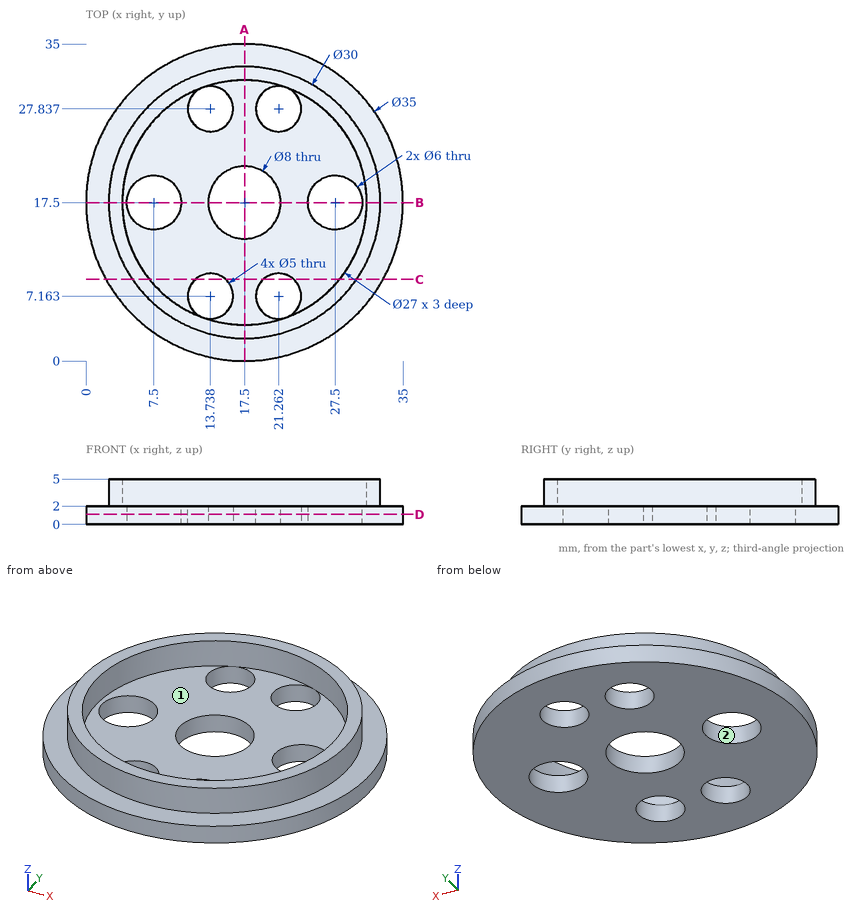
Design review of the part shown in the three views and the two pictorial views. Dimensions are in mm from the part's minimum x, y and z. A direction names the side the tool comes from. Round coordinates to 2 decimals unless told otherwise and drop trailing zeros. Loops run counter-clockwise (first coordinate to the right, second up) from the corner with the lowest first, then second, coordinate; pieces in that order, holes last. Notation, with made-up numbers: M -10,-19.5 L 23,-19.5 A37 ccw 23,17.5 Z; hole C 24,28.25 d5. An arc over 180 degrees is marked long. Answer as a JSON object with one key per item and string values.
Item 1: We need section D-D on z = 1.1. Give the boundary of the cut face in (x, y).
Answer sheet:
{"outline": "C 17.5,17.5 d35; hole C 7.5,17.5 d6; hole C 13.74,7.16 d5; hole C 13.74,27.84 d5; hole C 17.5,17.5 d8; hole C 21.26,7.16 d5; hole C 21.26,27.84 d5; hole C 27.5,17.5 d6"}
Item 2: Wall thickness on L1, parallel to X at y = 27, z = 0.65 (1 decimal); L2, parallel to Y at x = 22.5, z = 1.95 (1 decimal); L3, parallel to X at y = 7.5, z = 0.3 (1 decimal): over which ranges is each line inside the solid? List them lowest first. Write a range as from..to.
Answer sheet:
{"L1": "x = 2.8..11.4, 16.1..18.9, 23.6..32.2", "L2": "y = 0.7..5, 9.3..25.7, 30..34.3", "L3": "x = 3.1..11.3, 16.2..18.8, 23.7..31.9"}
Item 3: Machinability: for the marked faces 1 and 2, which of the approach directions +Z, -Z, +X, -X, +Y, -Y give a long, thin tool a straight path to every point of the face, cutting with its end or side? Answer none if there is none.
Answer sheet:
{"face 1": "+Z", "face 2": "+Z, -Z"}
Item 4: We need section B-B on y = 17.5. Give the boundary of the cut face in (x, z), and give its area (3 significant figures).
Answer sheet:
{"outline": "M 0,0 L 4.5,0 L 4.5,2 L 4,2 L 4,5 L 2.5,5 L 2.5,2 L 0,2 Z; M 10.5,0 L 13.5,0 L 13.5,2 L 10.5,2 Z; M 21.5,0 L 24.5,0 L 24.5,2 L 21.5,2 Z; M 30.5,0 L 35,0 L 35,2 L 32.5,2 L 32.5,5 L 31,5 L 31,2 L 30.5,2 Z", "area": "39.0 mm^2"}
Item 5: We need section A-A on x = 17.5. Give the boundary of the cut face in (y, z).
Answer sheet:
{"outline": "M 0,0 L 13.5,0 L 13.5,2 L 4,2 L 4,5 L 2.5,5 L 2.5,2 L 0,2 Z; M 21.5,0 L 35,0 L 35,2 L 32.5,2 L 32.5,5 L 31,5 L 31,2 L 21.5,2 Z"}
Item 6: We need section C-C on y = 9. Give the boundary of the cut face in (x, z).
Answer sheet:
{"outline": "M 2.2,0 L 12.04,0 L 12.04,2 L 7.01,2 L 7.01,5 L 5.14,5 L 5.14,2 L 2.2,2 Z; M 15.43,0 L 19.57,0 L 19.57,2 L 15.43,2 Z; M 22.96,0 L 32.8,0 L 32.8,2 L 29.86,2 L 29.86,5 L 27.99,5 L 27.99,2 L 22.96,2 Z"}
Item 7: Clearance check with flat-ended pins moving along their axes: P1, Ø4.5, axis at x = 21.26, y = 7.16, coming from the +Z side; P2, Ø6, axis at x = 24, y = 18, coming from the +Z side; P3, Ø1.5, axis at x = 31.5, z = 0.5, coming from the +Y side; P4, Ø1.5, axis at x = 30.5, z = 0.5, coming from the +Y side. State where each tip first meets the part, or that it passes through.
Answer sheet:
{"P1": "passes through", "P2": "stops at z = 2", "P3": "stops at y = 28.93", "P4": "stops at y = 30"}
